from build123d import *

# Parameters (mm, degrees)
CYLINDER003_R           = 2
CYLINDER003_DEPTH       = 30
CYLINDER003_PITCH_ANGLE = 90
CYLINDER002_R           = 2
CYLINDER002_DEPTH       = 30
CYLINDER002_PITCH_ANGLE = 90
BOX005_W                = 20
BOX005_H                = 20
BOX005_DEPTH            = 20


with BuildPart() as cylinder001:
    # Cylinder003 → Cylinder003 (new body)
    with BuildSketch(Plane.XY):
        Circle(CYLINDER003_R)
    extrude(amount=CYLINDER003_DEPTH)


with BuildPart() as cylinder001_1:
    # Cylinder003 pitch: moved
    add(cylinder001.part.rotate(Axis((0, 0, 0), (0, 1, 0)), CYLINDER003_PITCH_ANGLE))


with BuildPart() as cylinder001_2:
    # Cylinder003 placement: moved
    add(cylinder001_1.part.moved(Location((490, 313, 220))))


with BuildPart() as cylinder:
    # Cylinder002 → Cylinder002 (new body)
    with BuildSketch(Plane.XY):
        Circle(CYLINDER002_R)
    extrude(amount=CYLINDER002_DEPTH)


with BuildPart() as cylinder_1:
    # Cylinder002 pitch: moved
    add(cylinder.part.rotate(Axis((0, 0, 0), (0, 1, 0)), CYLINDER002_PITCH_ANGLE))


with BuildPart() as cylinder_2:
    # Cylinder002 placement: moved
    add(cylinder_1.part.moved(Location((490, 307, 220))))


with BuildPart() as plug001:
    # Box005 → Box005 (new body)
    with BuildSketch(Plane(origin=(485, 300, 210), x_dir=(1, 0, 0), z_dir=(0, 0, 1))):
        with Locations((10, 10)):
            Rectangle(BOX005_W, BOX005_H)
    extrude(amount=BOX005_DEPTH)

    # Cut001: cut Cylinder
    add(cylinder_2.part, mode=Mode.SUBTRACT)

    # Cut002: cut Cylinder001
    add(cylinder001_2.part, mode=Mode.SUBTRACT)


solid = plug001.part
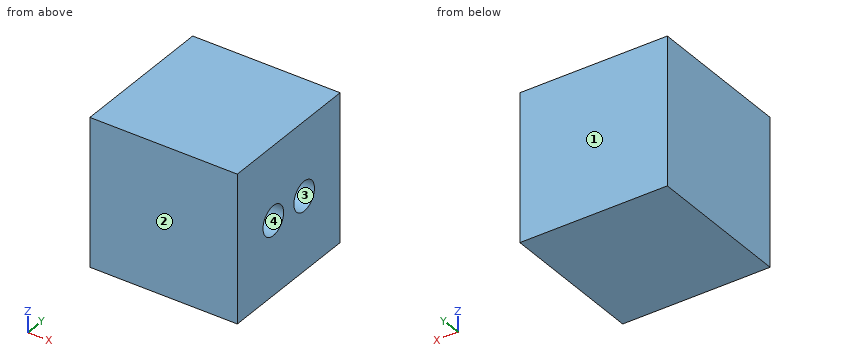
Geometry: final body of the model. Coordinates: model frame, mm. Face numbers are marked on the shaded views. Round coordinates to 2 decimals unless told otherwise and drop trailing zeros. Order: outer loops, then holes, each group sorted by start corner. A loop starts at its lowest first (then second) coordinate and runs counter-clockwise, first axis right, second up. Notation, with made-up numbers: (-24.75, 82.5) -> (34.25, 82.5) arc R24 ccw to (34.25, 110.5) -> close; hole circle Ø10 at (79.25, 73.5). An arc over 180 degrees is marked (long way). Put each result on its own line as item: value. Start each with the question number.
Q1. Section A-A on y = 313. Return the cut outline in (x, z).
Q2. Pull-direction query (Y, two-part tool) for the marked faces 1, 2, 3 and 4; classes: +Y half, -Y half, draft (parallel to the pull), parting line (faces both ways), or undercut.
Q3. First-contact query: pin 1 (3 mm diameter, centred on y = 313, z = 220, fed in from +X). Flat tip, straight axial feed; report the tip coordinate or a pass-through.
Q4. Section C-C on x = 495.25. Return the cut outline in (y, z).
Q5. Section B-B on z = 220. Return the cut outline in (x, y), and give its area (3 significant figures).
Q6. Line query: probe 1 along Y at (x, z) = (496.25, 220); probe 2 along Z at (x, y) = (500.5, 307); probe 3 along Y at (x, z) = (491.75, 221.25). Output: solid intervals per line, ascending.
Ans:
1. outline: (485, 210) -> (505, 210) -> (505, 218) -> (490, 218) -> (490, 222) -> (505, 222) -> (505, 230) -> (485, 230) -> close
2. face 1: +Y half
2. face 2: -Y half
2. face 3: undercut
2. face 4: undercut
3. pin 1: stops at x = 490
4. outline: (300, 210) -> (320, 210) -> (320, 230) -> (300, 230) -> close; hole circle Ø4 at (307, 220); hole circle Ø4 at (313, 220)
5. outline: (485, 300) -> (505, 300) -> (505, 305) -> (490, 305) -> (490, 309) -> (505, 309) -> (505, 311) -> (490, 311) -> (490, 315) -> (505, 315) -> (505, 320) -> (485, 320) -> close
5. area: 280 mm2
6. probe 1: y = 300 to 305, 309 to 311, 315 to 320
6. probe 2: z = 210 to 218, 222 to 230
6. probe 3: y = 300 to 305.44, 308.56 to 311.44, 314.56 to 320
